For this review, take the finished solid that the model builds, in its own axes (mm). A direction names the side the tool comes from. Give positions to 0.01 mm unless a question says otherwise; leave off trailing zeros. Order: outer loops, then holes, each group sorted by start corner. A loop starts at its lowest first (then second) coordinate and runs counter-clockwise, first axis right, second up.
from build123d import *

# Parameters (mm, degrees)
BOSS_EXTRUDE1_DEPTH = 5


with BuildPart() as part:
    # Sketch4 → Boss-Extrude1 (new, symmetric)
    with BuildSketch(Plane.XY):
        with BuildLine():
            Line((50, 40), (244.655381072, 40))
            ThreePointArc((244.655381072, 40), (351.936835728, 61.042418845), (443.320675573, 121.051482487))
            Line((443.320675573, 121.051482487), (459.066489093, 136.464981035))
            Line((459.066489093, 136.464981035), (494.796861895, 171.441265278))
            Line((494.796861895, 171.441265278), (522.777889288, 142.856967039))
            Line((522.777889288, 142.856967039), (487.047516486, 107.880682795))
            Line((487.047516486, 107.880682795), (471.305428262, 92.47083092))
            ThreePointArc((471.305428262, 92.47083092), (367.046513526, 24.007086549), (244.650168029, 0))
            Line((244.650168029, 0), (50, 0))
            Line((50, 0), (0, 0))
            Line((0, 0), (0, 40))
            Line((0, 40), (50, 40))
        make_face()
    extrude(amount=BOSS_EXTRUDE1_DEPTH, both=True)


solid = part.part
1) To check wall thickness, follow line 1 (Y direction, x = 107, z = 1); line 2 (Y direction, x = 251.5, z = -2.75); line 3 (X direction, y = 68, z = 1). State the ranges of each line that lie inside material, in increasing order.
Answer sheet:
line 1: y = 0 to 40
line 2: y = 0.07 to 40.08
line 3: x = 367.62 to 443.25
2) We need section A-A on z = 2. Give the boundary of the cut face in (x, y), then the cut area to 3 significant figures.
Answer sheet:
outline: (0, 0) - (244.65, 0) arc R324.01 ccw to (471.31, 92.47) - (522.78, 142.86) - (494.8, 171.44) - (443.32, 121.05) arc R284 cw to (244.66, 40) - (0, 40) - close
area: 22,100 mm2
3) We need section C-C on y = 103.5. Give the boundary of the cut face in (x, z), then the cut area to 3 significant figures.
Answer sheet:
outline: (423.64, -5) - (482.57, -5) - (482.57, 5) - (423.64, 5) - close
area: 589 mm2
4) Tool access review of faces 1 (the face through (0, 20, 0)), 2 (the face through (121, 40, 0)): name each direction out of +Z, -Z, +X, -X, +Y, -Y from which nothing blocks a thin tool from reaching the whole face with its end or side.
Answer sheet:
face 1: +Z, -Z, -X, +Y, -Y
face 2: +Z, -Z, -X, +Y
5) Clearance check with flat-ended pins moving along their axes: pin 1 (6 mm diameter, centred on x = 461, z = -3.5, fed in from +Y); pin 2 (1 mm diameter, centred on y = 129, z = 0, fed in from -X); pin 3 (4 mm diameter, centred on x = 226.5, z = -1.5, fed in from +Y). State where each tip first meets the part, or that it passes through.
Answer sheet:
pin 1: stops at y = 141.29
pin 2: stops at x = 450.93
pin 3: stops at y = 40
6) We need section B-B on x = 51.5. Give the boundary of the cut face in (y, z).
Answer sheet:
outline: (0, -5) - (40, -5) - (40, 5) - (0, 5) - close
